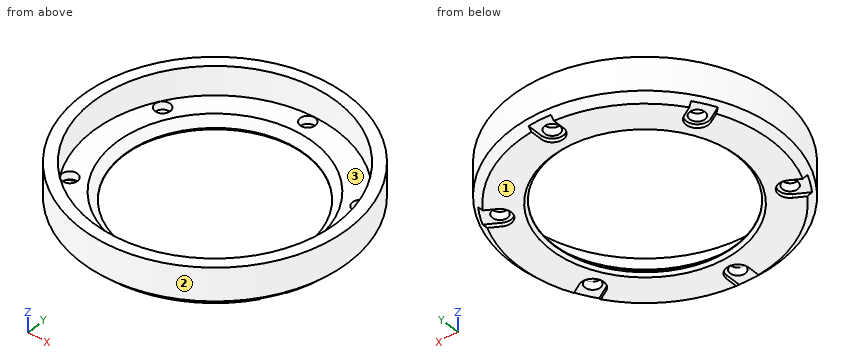
```python
from build123d import *

# Parameters (mm, degrees)
SKETCH1_R           = 18.5
BOSS_EXTRUDE1_DEPTH = 5.6
SHELL1_T            = -1.6
SKETCH2_R           = 12.6
CUT_EXTRUDE1_DEPTH  = 27.75556017
SKETCH3_R           = 1.05
CUT_EXTRUDE3_DEPTH  = 27.75556017
CIRPATTERN1_COUNT   = 6
CHAMFER1_SIZE       = 1
CUT_EXTRUDE4_DEPTH  = 0.5
CIRPATTERN2_COUNT   = 6
CHAMFER2_SIZE       = 0.4
CHAMFER3_SIZE       = 1.1


with BuildPart() as part:
    # Sketch1 → Boss-Extrude1 (new body)
    with BuildSketch(Plane.XY):
        Circle(SKETCH1_R)
    extrude(amount=BOSS_EXTRUDE1_DEPTH)

    # Shell1
    shell1_openings = [part.faces().sort_by_distance(p)[0] for p in [
        (0, 0, 5.6),
    ]]
    offset(amount=SHELL1_T, openings=shell1_openings, kind=Kind.INTERSECTION)

    # Sketch2 → Cut-Extrude1 (cut, through all)
    with BuildSketch(Plane(origin=(0, 0, 0), x_dir=(-1, 0, 0), z_dir=(0, 0, -1))):
        Circle(SKETCH2_R)
    extrude(amount=-CUT_EXTRUDE1_DEPTH, mode=Mode.SUBTRACT)

    # Sketch3 → Cut-Extrude3 (cut, through all)
    with BuildSketch(Plane.XY):
        with Locations((0, 15.8)):
            Circle(SKETCH3_R)
    cut_extrude3 = extrude(amount=CUT_EXTRUDE3_DEPTH, mode=Mode.SUBTRACT)

    # CirPattern1: Cut-Extrude3 ×6 about axis
    cirpattern1_axis = Axis((0, 0, 0), (0, 0, 1))
    for i in range(1, CIRPATTERN1_COUNT):
        add(cut_extrude3.rotate(cirpattern1_axis, i * 360 / CIRPATTERN1_COUNT), mode=Mode.SUBTRACT)

    # Chamfer1
    chamfer1_edges = [part.edges().sort_by_distance(p)[0] for p in [
        (-18.5, 0, 0),
    ]]
    chamfer(chamfer1_edges, length=CHAMFER1_SIZE)

    # Sketch4 → Cut-Extrude4 (cut)
    with BuildSketch(Plane(origin=(0, 0, 0), x_dir=(-1, 0, 0), z_dir=(0, 0, -1))):
        with BuildLine():
            Line((-1.55, -15.8), (-1.55, -18.667530629))
            Line((-1.55, -18.667530629), (1.55, -18.667530629))
            Line((1.55, -18.667530629), (1.55, -15.8))
            ThreePointArc((1.55, -15.8), (0, -14.25), (-1.55, -15.8))
        make_face()
    cut_extrude4 = extrude(amount=-CUT_EXTRUDE4_DEPTH, mode=Mode.SUBTRACT)

    # CirPattern2: Cut-Extrude4 ×6 about axis
    cirpattern2_axis = Axis((0, 0, 0), (0, 0, 1))
    for i in range(1, CIRPATTERN2_COUNT):
        add(cut_extrude4.rotate(cirpattern2_axis, i * 360 / CIRPATTERN2_COUNT), mode=Mode.SUBTRACT)

    # Chamfer2
    chamfer2_edges = [part.edges().sort_by_distance(p)[0] for p in [
        (12.6, 0, 0),
    ]]
    chamfer(chamfer2_edges, length=CHAMFER2_SIZE)

    # Chamfer3
    chamfer3_edges = [part.edges().sort_by_distance(p)[0] for p in [
        (12.6, 0, 1.6),
    ]]
    chamfer(chamfer3_edges, length=CHAMFER3_SIZE)


solid = part.part
```
Part model, mm, in its own coordinate system. Face numbers are marked on the shaded views. Round coordinates to 2 decimals unless told otherwise and drop trailing zeros. Use a Markdown table: item, result.
1) Probe line 1 (X direction, y = -0.5, z = 3.05); line 2 (Y direction, x = 0, z = 0.4); line 3 (Y direction, x = 0, z = 4.6). List the from-to ranges inside material, lowest first. Write a range as [from, to].
The answers:
| item | result |
|---|---|
| line 1 | x = [-18.49, -16.89], [16.89, 18.49] |
| line 2 | y = [-14.25, -12.6], [12.6, 14.25] |
| line 3 | y = [-18.5, -16.9], [16.9, 18.5] |
2) Drop flat-ended pins along their axis: pin 1 Ø12 at (x, y) = (4.5, 7) entering from +Z; pin 2 Ø1.6 at (x, y) = (0, 17) entering from -Z; pin 3 Ø1.3 at (x, y) = (-13.68, 7.9) entering from +Z; pin 4 Ø4.5 at (x, y) = (14.5, 7.5) entering from -Z. Give the stop position or say it passes through.
The answers:
| item | result |
|---|---|
| pin 1 | stops at z = 1.6 |
| pin 2 | stops at z = 0.5 |
| pin 3 | passes through |
| pin 4 | stops at z = 0 |
3) Pull direction X, two halves, no side cores. Call the marked faces 1, 2 and 3: pulls with the +X half, pulls with the -X half, needs draft (parallel to the pull), parting line crosses it, or undercut.
The answers:
| item | result |
|---|---|
| face 1 | needs draft |
| face 2 | parting line crosses it |
| face 3 | undercut |
4) Cut at A-A, the plane x = 0. State how many separate pieces and enclosed holes the cut face has, and give its area (3 significant figures).
The answers:
| item | result |
|---|---|
| separate pieces | 4 |
| enclosed holes | 0 |
| area | 21.2 mm2 |
